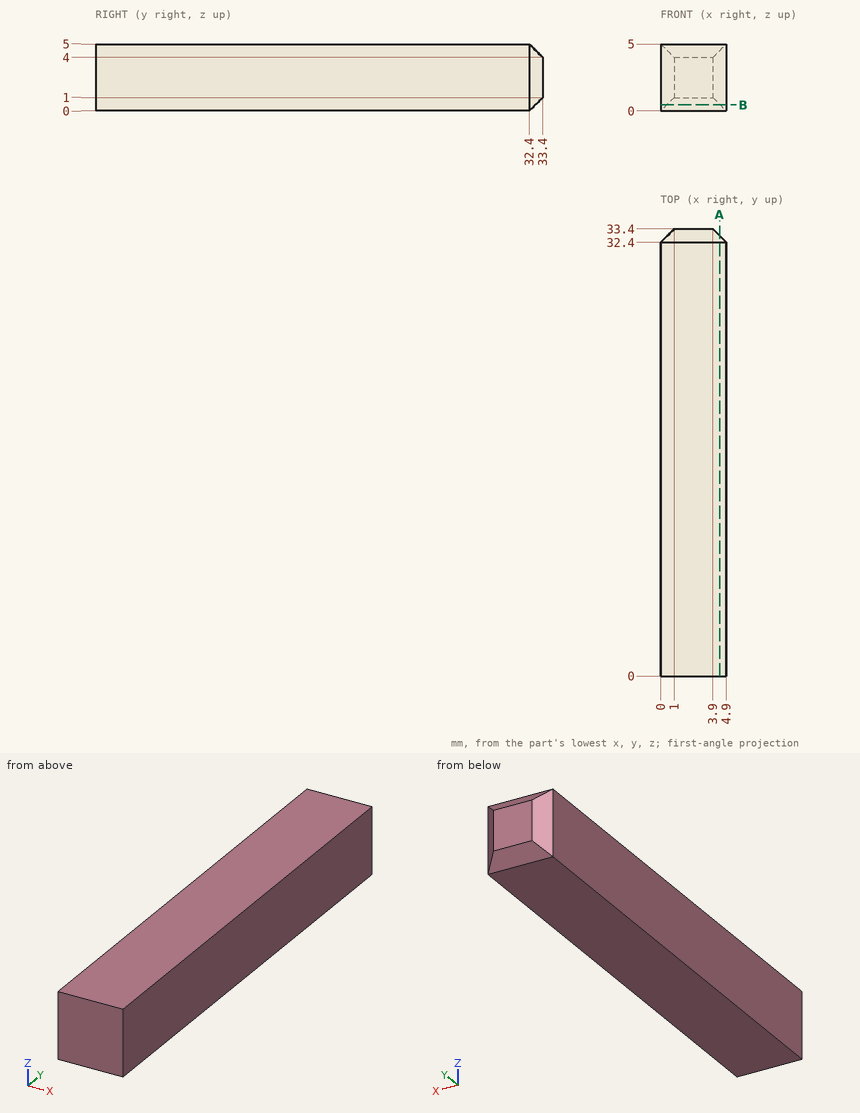
Verification items for this drawing (mm, ordinates from the low corner). Give positions to 0.01 mm unless a question says otherwise; leave off trailing zeros. Order: outer loops, then holes, each group sorted by start corner. A loop starts at its lowest first (then second) coordinate and runs counter-clockwise, first axis right, second up.
1) Cross-section at B-B (z = 0.45). Record the boundary of the cut face in (x, y), then the cut area to 3 significant figures.
Results are:
outline: (0, 0) - (4.9, 0) - (4.9, 32.4) - (4.45, 32.85) - (0.45, 32.85) - (0, 32.4) - close
area: 161 mm2
2) Cross-section at A-A (x = 4.4). Record the boundary of the cut face in (y, z), then the cut area to 3 significant figures.
Results are:
outline: (0, 0) - (32.4, 0) - (32.9, 0.5) - (32.9, 4.5) - (32.4, 5) - (0, 5) - close
area: 164 mm2
3) Material ranges on probe 1 along Y at (x, z) = (4.2, 4.35); probe 2 along Y at (x, z) = (4.6, 3.95); probe 3 along Z at (x, y) = (1.85, 32.5), recorded low to high.
Results are:
probe 1: y = 0 to 33.05
probe 2: y = 0 to 32.7
probe 3: z = 0.1 to 4.9
